Check sheet for the modelled part. Datum: model origin and axes. Units: mm. A direction names the side the tool comes from. Coordinates: 2 decimals unless noted, no trailing zeros. Order: outer loops, then holes, each group sorted by start corner. A loop starts at its lowest first (then second) coordinate and runs counter-clockwise, first axis right, second up. Notation, with made-up numbers: (-22.5, 77) -> (30.5, 77) arc R28 cw to (30.5, 99) -> close; hole circle Ø4 at (72, -24.75). An arc over 180 degrees is marked (long way). Put each result on its own line as item: value. Start each with the question number.
```python
from build123d import *

# Parameters (mm, degrees)
F0_W     = 44.45
F0_H     = 25.4
F1_DEPTH = 25.4
F2_W     = 31.75
F2_H     = 25.4
F3_DEPTH = 12.7
F4_W     = 12.7
F4_H     = 11.5118098885
F5_DEPTH = 6.35
F7_DEPTH = 12.7
F9_D     = 12.7


with BuildPart() as f1:
    # F0 (on Front) → F1 (new body)
    with BuildSketch(Plane.XZ):
        with Locations((22.225, 12.7)):
            Rectangle(F0_W, F0_H)
    extrude(amount=F1_DEPTH)

    # F2 (on face) → F3 (cut)
    with BuildSketch(Plane.XZ.offset(25.4)):
        with Locations((28.575, 12.7)):
            Rectangle(F2_W, F2_H)
    extrude(amount=-F3_DEPTH, mode=Mode.SUBTRACT)

    # F4 (on face) → F5 (cut)
    with BuildSketch(Plane.XZ.offset(25.4)):
        with Locations((6.35, 13.2940950558)):
            Rectangle(F4_W, F4_H)
    extrude(amount=-F5_DEPTH, mode=Mode.SUBTRACT)

    # F6 (on face) → F7 (cut, through all)
    with BuildSketch(Plane.XZ.offset(12.7)):
        with BuildLine():
            Line((44.45, 25.4), (22.8397343308, 25.4))
            ThreePointArc((22.8397343308, 25.4), (35.5397343308, 12.7), (22.8397343308, 0))
            Line((22.8397343308, 0), (44.45, 0))
            Line((44.45, 0), (44.45, 25.4))
        make_face()
    extrude(amount=-F7_DEPTH, mode=Mode.SUBTRACT)

    # F9 (through all)
    with Locations(Plane.XZ.offset(12.7)):
        with Locations((22.8397343308, 12.7)):
            Hole(F9_D / 2)


solid = f1.part
```
1) Sectioned sample at A-A (y = -22). Record the boundary of the cut face in (x, z).
2) Gauge pin test, flat ends, axial feed: pin 1 (9 mm diameter, centred on x = 9, z = 13.5, fed in from -Y); pin 2 (2 mm diameter, centred on x = 29.5, y = -3.5, fed in from -Z); pin 3 (10 mm diameter, centred on y = -21, z = 8, fed in from +X). Record the tip position at first contact, or that the pin passes through.
3) Sectioned sample at C-C (x = 3.5). Record the boundary of the cut face in (y, z), plus the area to 3 significant figures.
4) Sectioned sample at D-D (y = -9.5). Record the boundary of the cut face in (x, z).
5) Access from +Z, -Z, +X, -X, +Y, -Y to the whole of each face (thin tool, end or side, straight path). Record for faces 1 (the flat face through (26, -12.7, 19)), 2 (the flat face through (9, -10, 25.4)), 3 (the flat face through (6, -22, 7.538)).
6) Sectioned sample at B-B (z = 12.7). Record the boundary of the cut face in (x, y).
7) Scan lines: line 1 along X through (y, z) = (-14.75, 14); line 2 along Y through (x, z) = (29.5, 3.5); line 3 along Y through (x, z) = (8, 16). Record each from-to range of solid material in increasing order. Write a range as [from, to].
Entries:
1. outline: (0, 0) -> (12.7, 0) -> (12.7, 7.54) -> (0, 7.54) -> close; (0, 19.05) -> (12.7, 19.05) -> (12.7, 25.4) -> (0, 25.4) -> close
2. pin 1: stops at y = -19.05
2. pin 2: stops at z = 1.33
2. pin 3: stops at x = 12.7
3. outline: (-25.4, 0) -> (0, 0) -> (0, 25.4) -> (-25.4, 25.4) -> (-25.4, 19.05) -> (-19.05, 19.05) -> (-19.05, 7.54) -> (-25.4, 7.54) -> close
3. area: 572 mm2
4. outline: (0, 0) -> (22.84, 0) arc R12.7 ccw to (22.84, 25.4) -> (0, 25.4) -> close; hole circle Ø12.7 at (22.84, 12.7)
5. face 1: +Z, -Z, +X, -Y
5. face 2: +Z, +X, -X, +Y, -Y
5. face 3: +X, -X, -Y
6. outline: (0, -19.05) -> (12.7, -19.05) -> (12.7, -12.7) -> (16.49, -12.7) -> (16.49, 0) -> (0, 0) -> close; (29.19, -12.7) -> (35.54, -12.7) -> (35.54, 0) -> (29.19, 0) -> close
7. line 1: x = [0, 12.7]
7. line 2: y = [-12.7, 0]
7. line 3: y = [-19.05, 0]
